Geometry check sheet. Reference: the model listing, model coordinates, mm. Face numbers are marked on the shaded views. A direction names the side the tool comes from. Coordinates: 2 decimals unless noted, no trailing zeros. Write each loop counter-clockwise with the first axis right and the second up, starting at its lowest first coordinate (ties: lowest second). Pieces come first, ordered by that corner, then holes. Notation, with made-up numbers: (70.25, 21) -> (103.25, 21) arc R23 ccw to (103.25, 46) -> close; hole circle Ø6 at (10, 78.5). An arc over 180 degrees is marked (long way). Answer in a Markdown table with one row per item. Add a question column.
1. Set-up check for the marked faces 4 and 5: record each of +Z, -Z, +X, -X, +Y, -Y from which the full face is reachable in a straight line by a thin tool's end or side.
2. Mould release check, pull along X, two halves, no side actions. Record for the marked faces 1, 2 and 3: pulls with the +X half, pulls with the -X half, needs draft (parallel to the pull), parting line crosses it, or undercut.
3. Cross-section at A-A on x = 12.7. Record the cut outline in (y, z) (3 decimals).
4. Cross-section at B-B on z = -36.5. Record the cut outline in (x, y) (3 decimals).
5. Cross-section at D-D on z = -61. Record the cut outline in (x, y) (3 decimals).
6. Depth check by flat-ended pin: P1, Ø5, axis at x = 16.5, y = 19.5, coming from the -Z side (3 decimals). Enter the tip coordinate at first touch or a pass-through.
7. Scan lines: L1, parallel to Y at x = 12.7, z = -0.65; L2, parallel to Z at x = 2, y = 25.4 (3 decimals); L3, parallel to X at y = 28.5, z = -3.5 (3 decimals). Record each from-to range of solid material in increasing order. Write a range as from..to.
8. Cross-section at C-C on y = 23. Record the cut outline in (x, z) (3 decimals), and give its area (3 significant figures).
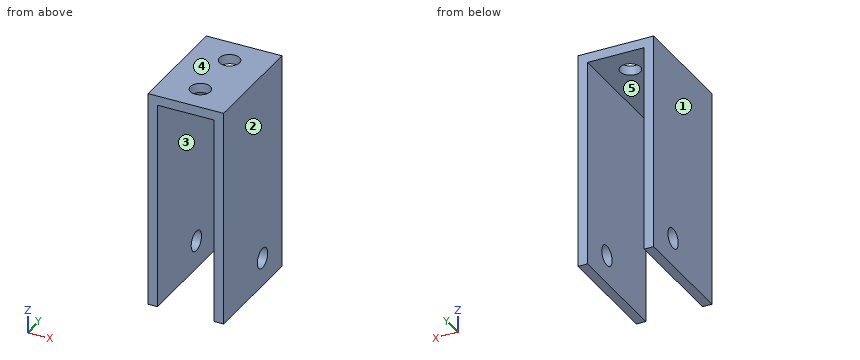
Autodesk Inventor part; units mm, degrees
ref_plane "YZ Plane" through (0, 0, 0) normal (1, 0, 0) x (0, 1, 0)
ref_plane "XZ Plane" through (0, 0, 0) normal (0, 1, 0) x (-1, 0, 0)
ref_plane "XY Plane" through (0, 0, 0) normal (0, 0, 1) x (1, 0, 0)
sketch "Sketch1" plane through (0, 0, 0) normal (0, 1, 0) x (-1, 0, 0)
  line L0 (0, 0) -> (0, -73.025)
  line L1 (0, -73.025) -> (-3.175, -73.025)
  line L2 (-3.175, -73.025) -> (-3.175, -3.175)
  line L3 (-3.175, -3.175) -> (-22.225, -3.175)
  line L4 (-22.225, -3.175) -> (-22.225, -73.025)
  line L5 (-22.225, -73.025) -> (-25.4, -73.025)
  line L6 (-25.4, -73.025) -> (-25.4, 0)
  line L7 (-25.4, 0) -> (0, 0)
  dimension "d0" = 3.175
  dimension "d1" = 73.025
  dimension "d2" = 3.175
  dimension "d3" = 25.4
  dimension "d4" = 3.175
extrude "Extrusion1" add sketch "Sketch1" along normal blind 38.1
sketch "Sketch2" plane through (25.4, 0, 0) normal (1, 0, 0) x (0, 0, -1)
  line L0 (73.025, 0) -> (73.025, 38.1)
  line L1 (73.025, 0) -> (0, 0)
  point P0 (63.5, 25.4)
  dimension "d7" = 9.525
  dimension "d8" = 25.4
hole "Hole1" at (25.4, 25.4, -63.5) direction (-1, 0, 0) diameter 6.7469 end through all
sketch "Sketch3" plane through (22.225, 0, -3.175) normal (0, 0, -1) x (-1, 0, 0)
  line L0 (-3.175, 0) -> (22.225, 0)
  line L1 (0, 38.1) -> (19.05, 38.1)
  line L2 (22.225, 0) -> (22.225, 38.1)
  line L3 (-3.175, 0) -> (-3.175, 38.1)
  point P0 (9.525, 9.525)
  point P1 (9.525, 28.575)
  point P2 (22.225, 31.75)
  point P3 (-3.175, 31.75)
  dimension "d19" = 9.525
  dimension "d20" = 9.525
  dimension "d21" = 12.7
  dimension "d22" = 12.7
hole "Hole2" at (12.7, 9.525, -3.175) at (12.7, 28.575, -3.175) direction (0, 0, 1) diameter 6.7469 end through all
properties part number "15102898-16-P-0311" material "Aluminum 6061"
Results found:
| question | item | result |
|---|---|---|
| 1 | face 4 | +Z, +X, -X, +Y, -Y |
| 1 | face 5 | -Z, +Y, -Y |
| 2 | face 1 | pulls with the -X half |
| 2 | face 2 | pulls with the +X half |
| 2 | face 3 | undercut |
| 3 | outline | (0, -3.175) -> (6.152, -3.175) -> (6.152, 0) -> (0, 0) -> close; (12.898, -3.175) -> (25.202, -3.175) -> (25.202, 0) -> (12.898, 0) -> close; (31.948, -3.175) -> (38.1, -3.175) -> (38.1, 0) -> (31.948, 0) -> close |
| 4 | outline | (0, 0) -> (3.175, 0) -> (3.175, 38.1) -> (0, 38.1) -> close; (22.225, 0) -> (25.4, 0) -> (25.4, 38.1) -> (22.225, 38.1) -> close |
| 5 | outline | (0, 0) -> (3.175, 0) -> (3.175, 23.135) -> (0, 23.135) -> close; (0, 27.665) -> (3.175, 27.665) -> (3.175, 38.1) -> (0, 38.1) -> close; (22.225, 0) -> (25.4, 0) -> (25.4, 23.135) -> (22.225, 23.135) -> close; (22.225, 27.665) -> (25.4, 27.665) -> (25.4, 38.1) -> (22.225, 38.1) -> close |
| 6 | P1 | stops at z = -3.175 |
| 7 | L1 | y = 0..6.15, 12.9..25.2, 31.95..38.1 |
| 7 | L2 | z = -73.025..-66.873, -60.127..0 |
| 7 | L3 | x = 0..3.175, 22.225..25.4 |
| 8 | outline | (0, -73.025) -> (3.175, -73.025) -> (3.175, -65.871) -> (0, -65.871) -> close; (0, -61.129) -> (3.175, -61.129) -> (3.175, -3.175) -> (22.225, -3.175) -> (22.225, -61.129) -> (25.4, -61.129) -> (25.4, 0) -> (0, 0) -> close; (22.225, -73.025) -> (25.4, -73.025) -> (25.4, -65.871) -> (22.225, -65.871) -> close |
| 8 | area | 494 mm^2 |
